Read the model definition and answer for the solid it produces. Units are mm, in the model's axes. A direction names the side the tool comes from. Coordinates: 2 decimals unless noted, no trailing zeros. Write each loop counter-clockwise with the first axis right and the second up, starting at its lowest first coordinate (ties: lowest second). Pieces come first, ordered by that corner, then holes. Notation, with made-up numbers: (-30.75, 21.25) -> (-4.75, 21.25) arc R26 cw to (-4.75, 48.25) -> close; hole circle Ø11 at (52.5, 56.25). An arc over 180 degrees is marked (long way). Use CSV: the item, a comma, the result in double quotes. Start each with the question number.
from build123d import *

# Parameters (mm, degrees)
CUT_EXTRUDE_3_DEPTH      = 73.537615195
CUT_EXTRUDE_3_DEPTH_BACK = 73.537615195
SKETCH_6_W               = 4.5
SKETCH_6_H               = 15
FILLET_1_R               = 6.8
SKETCH_4_R               = 2.15
CUT_EXTRUDE_1_DEPTH      = 74.261176759
SKETCH_5_R               = 2.15
CUT_EXTRUDE_2_DEPTH      = 74.261176759
PATTERN_LINEAR_1_COUNT   = 7
PATTERN_LINEAR_1_PITCH   = 8
FILLET_2_R               = 6.8
FILLET_3_R               = 1


with BuildPart() as part:
    # 草图2 → 放样1 section 0
    with BuildSketch(Plane(origin=(0, 70, 0), x_dir=(1, 0, 0), z_dir=(0, 1, 0))):
        with BuildLine():
            Line((-6.8, -16.8), (6.8, -16.8))
            Line((6.8, -16.8), (6.8, -3.2))
            Line((6.8, -3.2), (-6.8, -3.2))
            Line((-6.8, -3.2), (-6.8, -16.8))
        make_face()
    # 草图1 → 放样1 section 1
    with BuildSketch(Plane(origin=(0, 0, 0), x_dir=(1, 0, 0), z_dir=(0, 1, 0))):
        with BuildLine():
            Line((-6.8, -6.8), (6.8, -6.8))
            Line((6.8, -6.8), (6.8, 6.8))
            Line((6.8, 6.8), (-6.8, 6.8))
            Line((-6.8, 6.8), (-6.8, -6.8))
        make_face()
    loft()

    # 草图6 → 切除-拉伸3 (cut, two sides: drawn at the far end of the back side and taken through both)
    with BuildSketch(Plane(origin=(0, -0.952, 6.664), x_dir=(1, 0, 0), z_dir=(0, -0.14142135623730942, 0.9899494936611666)).offset(-CUT_EXTRUDE_3_DEPTH_BACK)):
        with Locations((0, 64.172343341)):
            Rectangle(SKETCH_6_W, SKETCH_6_H)
    extrude(amount=CUT_EXTRUDE_3_DEPTH + CUT_EXTRUDE_3_DEPTH_BACK, mode=Mode.SUBTRACT)

    # 圆角1
    fillet_1_edges = [part.edges().sort_by_distance(p)[0] for p in [
        (4.525, 70, 3.2),
        (-4.525, 70, 16.8),
    ]]
    fillet(fillet_1_edges, radius=FILLET_1_R)

    # 草图4 → 切除-拉伸1 (cut, through all)
    with BuildSketch(Plane(origin=(6.8, 0, 0), x_dir=(0, 0, -1), z_dir=(1, 0, 0))):
        with Locations(Location((-8.967347222, 63, 0), (0, 0, 270))):
            Circle(SKETCH_4_R)
    extrude(amount=-CUT_EXTRUDE_1_DEPTH, mode=Mode.SUBTRACT)

    # 草图5 → 切除-拉伸2 (cut, through all)
    with BuildSketch(Plane(origin=(6.8, 0, 0), x_dir=(0, 0, -1), z_dir=(1, 0, 0))):
        with Locations(Location((-0.711694224, 5, 0), (0, 0, 90))):
            Circle(SKETCH_5_R)
    cut_extrude_2 = extrude(amount=-CUT_EXTRUDE_2_DEPTH, mode=Mode.SUBTRACT)

    # 阵列(线性)1: 切除-拉伸2 ×7
    with Locations(*[Vector(0, 0.9899494936611666, 0.14142135623730945) * (i * PATTERN_LINEAR_1_PITCH) for i in range(1, PATTERN_LINEAR_1_COUNT)]):
        add(cut_extrude_2, mode=Mode.SUBTRACT)

    # 圆角2
    # the kernel refuses this fillet: 6.8 mm, written as the material it takes off along each edge
    with BuildSketch(Plane(origin=(12.490471053, 70, 3.2), x_dir=(0, -0.9899494936611667, -0.14142135623730884), z_dir=(-1, 0, 0))) as fillet_2_piece_1:
        with BuildLine():
            CenterArc((5.896188421, 6.8), FILLET_2_R, 189.295271006, 80.704728994)
            Line((-0.814521127, 5.701647891), (-0.948735318, 5.679680849))
            ThreePointArc((-0.948735318, 5.679680849), (-0.541893695, 2.831590641), (-0.134633131, -0.019233304))
            Line((-0.134633131, -0.019233304), (0, -0.136))
            Line((0, -0.136), (5.896188421, -0.136))
            Line((5.896188421, -0.136), (5.896188421, 0))
        make_face()
    extrude(amount=34.030942106, mode=Mode.SUBTRACT)
    with BuildSketch(Plane(origin=(-17.347634455, 70, 16.8), x_dir=(0, -0.9899494936611665, -0.14142135623730936), z_dir=(1, 0, 0))) as fillet_2_piece_2:
        with BuildLine():
            CenterArc((7.839053782, 6.8), FILLET_2_R, 173.031690524, 96.968309476)
            Line((1.089282619, 7.624978336), (0.954287196, 7.641477903))
            ThreePointArc((0.954287196, 7.641477903), (0.410008179, 3.831722473), (-0.134633131, 0.019233304))
            Line((-0.134633131, 0.019233304), (0, -0.136))
            Line((0, -0.136), (7.839053782, -0.136))
            Line((7.839053782, -0.136), (7.839053782, 0))
        make_face()
    extrude(amount=43.745268909, mode=Mode.SUBTRACT)

    # 圆角3
    fillet_3_edges = [part.edges().sort_by_distance(p)[0] for p in [
        (0, 0, -6.8),
        (6.8, 0, 0),
        (0, 0, 6.8),
    ]]
    fillet(fillet_3_edges, radius=FILLET_3_R)


solid = part.part
1) Find the intervals of material crossed by line 1 along X through (y, z) = (59, 3.75); line 2 along Y through (x, z) = (5, 4.75); line 3 along Y through (x, z) = (4, 6.75), in increasing order.
2) The mould has two halves that part along Z. Classify faces 3 (the face through (4.49, 68.38, 4.69)), 4 (the face through (0, 0, 0)), 5 (the face through (0.1, 42.45, 6.46)): pulls with the +Z half, pulls with the -Z half, needs draft (parallel to the pull), parting line crosses it, or undercut.
3) Section B-B, the plane x = 0.5 is taken. Give the vertices of the cut face in (y, z).
4) Section A-A, the plane x = 4.5 is taken. Count the separate pieces of the cut face and the enclosed holes in it, plus the area to 3 significant figures.
5) Each of these flat-tipped pins is pushed along its axis until it touches: pin 1 (3 mm diameter, centred on x = -1.5, y = 45, fed in from -Z); pin 2 (3 mm diameter, centred on x = -3, y = 24.5, fed in from +Z); pin 3 (4 mm diameter, centred on x = 4, z = 12.5, fed in from +Y). Where does it stop, or does it pass through?
6) Which of the six approach directions +Z, -Z, +X, -X, +Y, -Y give full straight-line access (tool end or side, diameter ignored) to faces 1 (the face through (-0.031, 56.116, 7.921)), 2 (the face through (-4.5, 68.3, 4.6))?
The answers:
1,line 1,"x = -6.8 to -2.25, 2.25 to 6.8"
1,line 2,"y = 0 to 19.63, 22.05 to 26.71, 30.81 to 34.58, 38.77 to 43.18, 46.01 to 68.43"
1,line 3,"y = 0.42 to 35.15, 38.21 to 42.48, 46.71 to 50.5, 54.53 to 69.58"
2,face 3,"pulls with the -Z half"
2,face 4,"needs draft"
2,face 5,"undercut"
3,outline,"(0, -5.65) arc R1 ccw to (1.14, -6.64) -> (57.05, 1.35) -> (55.15, 14.68) -> (0.86, 6.92) arc R1 ccw to (0, 5.93) -> close; hole circle Ø4.3 at (5, 0.71); hole circle Ø4.3 at (12.92, 1.84); hole circle Ø4.3 at (20.84, 2.97); hole circle Ø4.3 at (28.76, 4.11); hole circle Ø4.3 at (36.68, 5.24); hole circle Ø4.3 at (44.6, 6.37); hole circle Ø4.3 at (52.52, 7.5)"
4,separate pieces,"1"
4,enclosed holes,"8"
4,area,"815 mm^2"
5,pin 1,"stops at z = -0.59"
5,pin 2,"stops at z = 10.51"
5,pin 3,"stops at y = 69.82"
6,face 1,"+Z, +Y"
6,face 2,"-Z, +X, -X, +Y"
